from build123d import *

# Parameters (mm, degrees)
F0_R        = 25.6
F0_R_2      = 1.5
F1_DEPTH    = 3
F2_COUNT    = 5
F3_T1_DEPTH = 3
F4_R        = 2


# Not quite as in the source:
# - a fillet or chamfer that OpenCascade refuses, or shapes differently, is made with other operations: its cross-section is extruded or revolved along the edge and cut away or added


with BuildPart() as f1:
    # F0 (on Front) → F1 (new body)
    with BuildSketch(Plane.XZ):
        Circle(F0_R)
        with BuildLine():
            ThreePointArc((-1.4990055262, 20.5453883495), (0, 20.6), (1.4990055262, 20.5453883495))
            ThreePointArc((1.4990055262, 20.5453883495), (15.0870725099, 14.0264123382), (20.6, 0))
            ThreePointArc((20.6, 0), (-14.0264123382, -15.0870725099), (-1.4990055262, 20.5453883495))
        make_face(mode=Mode.SUBTRACT)
        with BuildLine():
            ThreePointArc((-1.9720265944, 5.6666666667), (-3.4761933515, -4.8904069139), (6, 0))
            ThreePointArc((6, 0), (4.8904069139, 3.4761933515), (1.9720265944, 5.6666666667))
            ThreePointArc((1.9720265944, 5.6666666667), (0, 6), (-1.9720265944, 5.6666666667))
        make_face()
        Circle(F0_R_2, mode=Mode.SUBTRACT)
        with BuildLine():
            ThreePointArc((-1.9720265944, 5.6666666667), (0, 6), (1.9720265944, 5.6666666667))
            Line((1.9720265944, 5.6666666667), (1.4990055262, 20.5453883495))
            ThreePointArc((1.4990055262, 20.5453883495), (0, 20.6), (-1.4990055262, 20.5453883495))
            Line((-1.4990055262, 20.5453883495), (-1.9720265944, 5.6666666667))
        make_face()
    extrude(amount=F1_DEPTH)

    # F2: F1 ×5 about axis
    f2_axis = Axis((0, 0, 0), (0, -1, 0))


with BuildPart() as f1_1:
    add(f1.part)
    for i in range(1, F2_COUNT):
        add(f1.part.rotate(f2_axis, i * 360 / F2_COUNT))

    # F3: fillet of radius 5.08 on 10 edges, made by hand

    # F3_s2 → F3_t1 (join)
    with BuildSketch(Plane.XZ):
        with BuildLine():
            ThreePointArc((1.8832465894, 8.4592124416), (2.4124774845, 6.3578379743), (3.7693220099, 4.6682128899))
            ThreePointArc((3.7693220099, 4.6682128899), (2.9137601883, 5.244997766), (1.9720265944, 5.6666666667))
            Line((1.9720265944, 5.6666666667), (1.8832465894, 8.4592124416))
        make_face()
        with BuildLine():
            ThreePointArc((3.2749497301, 5.0273953759), (5.3011666938, 4.2590824136), (7.4632339146, 4.4051143441))
            Line((7.4632339146, 4.4051143441), (4.779930528, 3.6266050443))
            ThreePointArc((4.779930528, 3.6266050443), (4.0878878875, 4.3919440592), (3.2749497301, 5.0273953759))
        make_face()
        with BuildLine():
            ThreePointArc((5.7933522546, -1.5611116727), (5.6887786813, -3.7255802818), (6.4957788146, -5.7367020526))
            Line((6.4957788146, -5.7367020526), (4.9261861245, -3.4253014855))
            ThreePointArc((4.9261861245, -3.4253014855), (5.440213845, -2.5306270607), (5.7933522546, -1.5611116727))
        make_face()
        with BuildLine():
            ThreePointArc((-3.7693220099, 4.6682128899), (-2.4124774845, 6.3578379743), (-1.8832465894, 8.4592124416))
            Line((-1.8832465894, 8.4592124416), (-1.9720265944, 5.6666666667))
            ThreePointArc((-1.9720265944, 5.6666666667), (-2.9137601883, 5.244997766), (-3.7693220099, 4.6682128899))
        make_face()
        with BuildLine():
            ThreePointArc((-7.4632339146, 4.4051143441), (-5.3011666938, 4.2590824136), (-3.2749497301, 5.0273953759))
            ThreePointArc((-3.2749497301, 5.0273953759), (-4.0878878875, 4.3919440592), (-4.779930528, 3.6266050443))
            Line((-4.779930528, 3.6266050443), (-7.4632339146, 4.4051143441))
        make_face()
        with BuildLine():
            ThreePointArc((-5.6045188467, -2.1422811432), (-6.7921597763, -0.3297224505), (-8.627144316, 0.8229664629))
            Line((-8.627144316, 0.8229664629), (-5.99870999, -0.1244124414))
            ThreePointArc((-5.99870999, -0.1244124414), (-5.888690719, -1.1503571689), (-5.6045188467, -2.1422811432))
        make_face()
        with BuildLine():
            ThreePointArc((-6.4957788146, -5.7367020526), (-5.6887786813, -3.7255802818), (-5.7933522546, -1.5611116727))
            ThreePointArc((-5.7933522546, -1.5611116727), (-5.440213845, -2.5306270607), (-4.9261861245, -3.4253014855))
            Line((-4.9261861245, -3.4253014855), (-6.4957788146, -5.7367020526))
        make_face()
        with BuildLine():
            ThreePointArc((0.3055388721, -5.9922154499), (-1.7853081143, -6.5616176556), (-3.4486218238, -7.950591196))
            Line((-3.4486218238, -7.950591196), (-1.7353800681, -5.7435577841))
            ThreePointArc((-1.7353800681, -5.7435577841), (-0.7256508252, -5.9559575955), (0.3055388721, -5.9922154499))
        make_face()
        with BuildLine():
            ThreePointArc((3.4486218238, -7.950591196), (1.7853081143, -6.5616176556), (-0.3055388721, -5.9922154499))
            ThreePointArc((-0.3055388721, -5.9922154499), (0.7256508252, -5.9559575955), (1.7353800681, -5.7435577841))
            Line((1.7353800681, -5.7435577841), (3.4486218238, -7.950591196))
        make_face()
        with BuildLine():
            ThreePointArc((8.627144316, 0.8229664629), (6.7921597763, -0.3297224505), (5.6045188467, -2.1422811432))
            ThreePointArc((5.6045188467, -2.1422811432), (5.888690719, -1.1503571689), (5.99870999, -0.1244124414))
            Line((5.99870999, -0.1244124414), (8.627144316, 0.8229664629))
        make_face()
    extrude(amount=F3_T1_DEPTH)

    # F4
    f4_edges = [f1_1.edges().sort_by_distance(p)[0] for p in [
        (1.499006, -1.5, 20.545388),
        (-20.003044, -1.5, 4.923235),
        (20.003044, -1.5, 4.923235),
        (10.863555, -1.5, -17.502662),
        (-1.499006, -1.5, 20.545388),
        (19.076607, -1.5, 7.774513),
        (13.288997, -1.5, -15.740475),
        (-19.076607, -1.5, 7.774513),
        (-10.863555, -1.5, -17.502662),
        (-13.288997, -1.5, -15.740475),
    ]]
    fillet(f4_edges, radius=F4_R)


solid = f1_1.part
CAD build for the part. Positions are in the model's coordinates, mm. A direction names the side the tool comes from. Round coordinates to 2 decimals unless told otherwise and drop trailing zeros. Write each loop counter-clockwise with the first axis right and the second up, starting at its lowest first coordinate (ties: lowest second). Pieces come first, ordered by that corner, then holes.
(1) Slice it at A-A, the plane x = -2.5. Write the cut outline in (y, z).
(2) Probe line 1 along X through (y, z) = (-0.7, 0); line 2 along X through (y, z) = (-1.8, -2); line 3 along X through (y, z) = (-1.25, -8). List the from-to ranges inside material, lowest first.
(3) 3-axis set-ups, long thin cutter, end or side, ignore diameter. For faces 5 (the face through (0, 0, -5)), 6 (the face through (2.334, -1.479, 6.522)): which of +Z, -Z, +X, -X, +Y, -Y reach the whole face in a straight line?
(4) Slice it at B-B, the plane y = -2.2. Count the separate pieces of the cut face and the enclosed holes in it, and give its area (3 significant figures).
(5) Mould opens along X. For faces 1 (the face through (-20.3, -1.5, -15.6)), 2 (the face through (0, -3, -5)), 3 (the face through (-5.481, -1.479, 4.236)), 4 (the face through (6.39, -1.48, -11.74)) say: pulls with the +X half, pulls with the -X half, needs draft (parallel to the pull), parting line crosses it, or undercut.
From the geometry:
1. outline: (-3, -25.48) - (0, -25.48) - (0, -20.45) - (-3, -20.45) - close; (-3, -7.01) - (0, -7.01) - (0, 6.19) - (-3, 6.19) - close; (-3, 19.94) - (0, 19.94) - (0, 25.48) - (-3, 25.48) - close
2. line 1: x = -25.6 to -20.6, -7.16 to -1.5, 1.5 to 7.16, 20.6 to 25.6
2. line 2: x = -25.52 to -20.5, -5.7 to 5.7, 20.5 to 25.52
2. line 3: x = -24.32 to -18.98, -8.03 to -3.49, 3.49 to 8.03, 18.98 to 24.32
3. face 5: +Z, -Z, +X, -X, +Y
3. face 6: +Y, -Y
4. separate pieces: 1
4. enclosed holes: 6
4. area: 1,110 mm2
5. face 1: parting line crosses it
5. face 2: needs draft
5. face 3: undercut
5. face 4: undercut
